```python
from build123d import *

# Parameters (mm, degrees)
SKETCH1_R      = 12.7
SKETCH1_R_2    = 5.461
EXTRUDE1_DEPTH = 25.4
SKETCH2_R      = 19.05
SKETCH2_R_2    = 5.461
EXTRUDE2_DEPTH = 127
SKETCH5_R      = 34.671
SKETCH5_R_2    = 12.7
EXTRUDE3_DEPTH = 12.7
SKETCH7_R      = 37.719
EXTRUDE4_DEPTH = 19.05
SKETCH9_R      = 28.575
EXTRUDE6_DEPTH = 97.79
SKETCH10_R     = 14.187120342
EXTRUDE7_DEPTH = 38.354
SKETCH11_R     = 34.925
EXTRUDE8_DEPTH = 12.7
SKETCH12_R     = 5.461
EXTRUDE9_DEPTH = 153.4


with BuildPart() as part:
    # Sketch1 → Extrude1 (new body)
    with BuildSketch(Plane(origin=(0, 0, 0), x_dir=(1, 0, 0), z_dir=(0, 1, 0))):
        Circle(SKETCH1_R)
        Circle(SKETCH1_R_2, mode=Mode.SUBTRACT)
    extrude(amount=EXTRUDE1_DEPTH)

    # Sketch2 → Extrude2 (add)
    with BuildSketch(Plane(origin=(0, 25.4, 0), x_dir=(1, 0, 0), z_dir=(0, 1, 0))):
        Circle(SKETCH2_R)
        Circle(SKETCH2_R_2, mode=Mode.SUBTRACT)
    extrude(amount=EXTRUDE2_DEPTH)

    # Sketch5 → Extrude3 (add)
    with BuildSketch(Plane.XZ):
        Circle(SKETCH5_R)
        Circle(SKETCH5_R_2, mode=Mode.SUBTRACT)
    extrude(amount=-EXTRUDE3_DEPTH)



with BuildPart() as body_2:
    # Sketch7 → Extrude4 (new body)
    with BuildSketch(Plane(origin=(0, 106.68136068, -61.21263932), x_dir=(-1, 0, 0), z_dir=(0, -0.707106781, 0.707106781))):
        Circle(SKETCH7_R)
    extrude(amount=EXTRUDE4_DEPTH)


with BuildPart() as part_1:
    add(part.part)

    add(body_2.part)  # Extrude6 merges body 2
    # Sketch9 → Extrude6 (add)
    with BuildSketch(Plane(origin=(0, 83.947, -83.947), x_dir=(1, 0, 0), z_dir=(0, 0.707106781, -0.707106781))):
        with Locations((0, -32.151241205)):
            Circle(SKETCH9_R)
    extrude(amount=-EXTRUDE6_DEPTH)

    # Sketch10 → Extrude7 (add)
    with BuildSketch(Plane(origin=(0, 83.947, -83.947), x_dir=(1, 0, 0), z_dir=(0, 0.707106781, -0.707106781))):
        with Locations((0, -32.151241205)):
            Circle(SKETCH10_R)
    extrude(amount=EXTRUDE7_DEPTH)

    # Sketch11 → Extrude8 (add)
    with BuildSketch(Plane(origin=(0, 152.4, 0), x_dir=(1, 0, 0), z_dir=(0, 1, 0))):
        Circle(SKETCH11_R)
    extrude(amount=-EXTRUDE8_DEPTH)

    # Sketch12 → Extrude9 (cut, through all)
    with BuildSketch(Plane.XZ):
        Circle(SKETCH12_R)
    extrude(amount=-EXTRUDE9_DEPTH, mode=Mode.SUBTRACT)


solid = part_1.part
```
The model under review builds one solid part; all positions refer to its coordinate system, in mm. A direction names the side the tool comes from. Round coordinates to 2 decimals unless told otherwise and drop trailing zeros. Order: outer loops, then holes, each group sorted by start corner. A loop starts at its lowest first (then second) coordinate and runs counter-clockwise, first axis right, second up. Notation, with made-up numbers: (-23.75, 34.25) - (17.25, 34.25) arc R36 ccw to (17.25, 68.25) - close; hole circle Ø11 at (-10.5, 60.5). An arc over 180 degrees is marked (long way). Answer in a Markdown table with one row per item.
(1) Take a section at C-C on z = -32. Count the separate pieces of the cut face and the enclosed holes in it, plus the area to 3 significant figures.
Result set:
| item | result |
|---|---|
| separate pieces | 3 |
| enclosed holes | 0 |
| area | 5,040 mm2 |
(2) Machinability: for faces 1 (the face through (-0.199, 133.661, -88.473)), 2 (the face through (-27.715, 146.139, 21.251)), 3 (the face through (15, 139.7, 15)), which of the approach directions +Z, -Z, +X, -X, +Y, -Y give a long, thin tool a straight path to every point of the face, cutting with its end or side? Answer none if there is none.
Result set:
| item | result |
|---|---|
| face 1 | -Z, +X, -X, +Y |
| face 2 | +Y |
| face 3 | none |
(3) For line 1 (X direction, y = 91.5, z = 0); line 2 (Y direction, x = -6, z = -31); line 3 (X direction, y = 15, z = 0), list the stretches that pass through material, from the lowest coordinate up. Write a range as from..to.
Result set:
| item | result |
|---|---|
| line 1 | x = -19.05..-5.46, 5.46..19.05 |
| line 2 | y = 0..12.7, 36.96..129.13, 139.7..152.4 |
| line 3 | x = -12.7..-5.46, 5.46..12.7 |
(4) Clearance check with flat-ended pins moving along their axes: P1, Ø1.5, axis at x = 14.5, y = 66, coming from the +Z side; P2, Ø12, axis at y = 62.5, z = 19, coming from the -X side; P3, Ø2, axis at x = 24, z = -75, coming from the +Y side. State where each tip first meets the part, or that it passes through.
Result set:
| item | result |
|---|---|
| P1 | stops at z = 15.26 |
| P2 | stops at x = -20.91 |
| P3 | stops at y = 93.89 |
(5) Take a section at B-B on x = -22.5. Write out the cut boundary in (y, z), plus the area to 3 significant figures.
Result set:
| item | result |
|---|---|
| outline | (0, -26.38) - (12.7, -26.38) - (12.7, 26.38) - (0, 26.38) - close; (25.08, -4.52) - (80.76, -60.2) - (71.8, -69.15) - (85.27, -82.62) - (128.09, -39.81) - (114.62, -26.34) - (105.67, -35.29) - (49.99, 20.39) - close; (139.7, -26.71) - (152.4, -26.71) - (152.4, 26.71) - (139.7, 26.71) - close |
| area | 5,280 mm2 |
(6) Mouldability with a two-part tool opening along Y and no side actions: class faces 4 (the face through (7, 0, 0)), 5 (the face through (7.627, 111.593, -83.042)), 6 (the face through (-34.637, 6.261, 1.524)) as released by +Y, released by -Y, zero draft, split by the parting line, or undercut.
Result set:
| item | result |
|---|---|
| face 4 | released by -Y |
| face 5 | undercut |
| face 6 | zero draft |
